from build123d import *

# Parameters (mm, degrees)
F1_DEPTH = 12
F2_DEPTH = 7


# Not quite as in the source:
# - a feature of the source that left no trace in its solid (it failed there, or was rolled back) is left out


with BuildPart() as f1:
    # F0 (on Front) → F1 (new body)
    with BuildSketch(Plane.XZ):
        with BuildLine():
            Line((70, 130), (70, 230))
            ThreePointArc((70, 230), (0, 300), (-70, 230))
            Line((-70, 230), (-70, 130))
            ThreePointArc((-70, 130), (0, 60), (70, 130))
        make_face()
        with BuildLine():
            Line((-65, 130), (-65, 230))
            ThreePointArc((-65, 230), (0, 295), (65, 230))
            Line((65, 230), (65, 130))
            ThreePointArc((65, 130), (0, 65), (-65, 130))
        make_face(mode=Mode.SUBTRACT)
        with BuildLine():
            ThreePointArc((65, 230), (0, 295), (-65, 230))
            Line((-65, 230), (-65, 130))
            ThreePointArc((-65, 130), (0, 65), (65, 130))
            Line((65, 130), (65, 230))
        make_face()
        with BuildLine():
            Line((-50, 130), (-50, 230))
            ThreePointArc((-50, 230), (0, 280), (50, 230))
            Line((50, 230), (50, 130))
            ThreePointArc((50, 130), (0, 80), (-50, 130))
        make_face(mode=Mode.SUBTRACT)
    extrude(amount=F1_DEPTH)

    # F0 (on Front) → F2 (cut)
    with BuildSketch(Plane.XZ):
        with BuildLine():
            ThreePointArc((65, 230), (0, 295), (-65, 230))
            Line((-65, 230), (-65, 130))
            ThreePointArc((-65, 130), (0, 65), (65, 130))
            Line((65, 130), (65, 230))
        make_face()
        with BuildLine():
            Line((-50, 130), (-50, 230))
            ThreePointArc((-50, 230), (0, 280), (50, 230))
            Line((50, 230), (50, 130))
            ThreePointArc((50, 130), (0, 80), (-50, 130))
        make_face(mode=Mode.SUBTRACT)
    extrude(amount=F2_DEPTH, mode=Mode.SUBTRACT)


solid = f1.part
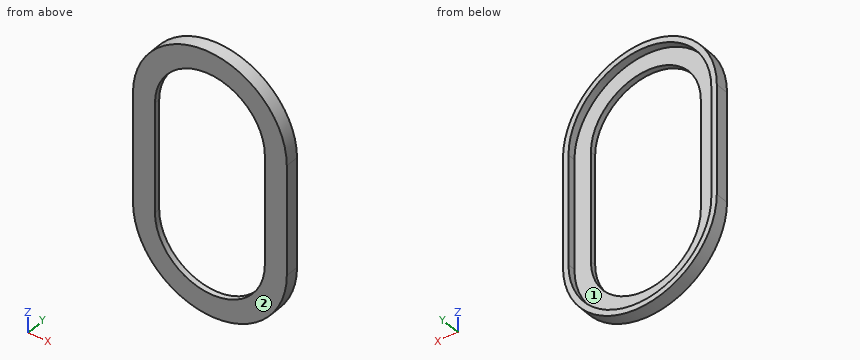
Geometry check sheet. Reference: the model listing, model coordinates, mm. Face numbers are marked on the shaded views. A direction names the side the tool comes from. Round coordinates to 2 decimals unless told otherwise and drop trailing zeros. Order: outer loops, then holes, each group sorted by start corner. A loop starts at its lowest first (then second) coordinate and runs counter-clockwise, first axis right, second up. Notation, with made-up numbers: (63.5, 19.25) -> (94.5, 19.25) arc R12 ccw to (94.5, 26.25) -> close; hole circle Ø2 at (11, 84.25). An arc over 180 degrees is marked (long way). Use one line per item in the form item = value.
1. Cross-section at C-C, the plane x = -56. Enter the section's corners in (y, z), plus the area to 3 significant figures.
Working result:
outline = (-12, 88) -> (0, 88) -> (0, 97) -> (-7, 97) -> (-7, 263) -> (0, 263) -> (0, 272) -> (-12, 272) -> close
area = 1,050 mm^2
2. Go/stop test with flat-tipped pins: pin 1 (6 mm diameter, centred on x = 35.5, y = -2, fed in from -Z); pin 2 (4 mm diameter, centred on y = -8, z = 258, fed in from -X); pin 3 (10 mm diameter, centred on x = -48.5, z = 128, fed in from +Y). Record where each tip stops, or that it passes through.
Working result:
pin_1 = 68
pin_2 = -64.99
pin_3 = -7
3. Scan lines: line 1 along X through (y, z) = (-0.5, 173); line 2 along X through (y, z) = (-9.5, 138.5); line 3 along Y through (x, z) = (57, 141.5). Record each from-to range of solid material in increasing order. Write a range as from..to.
Working result:
line_1 = -70..-65, 65..70
line_2 = -70..-50, 50..70
line_3 = -12..-7
4. Set-up check for the marked faces 1 and 2: record each of +Z, -Z, +X, -X, +Y, -Y from which the full face is reachable in a straight line by a thin tool's end or side.
Working result:
face_1 = +Y
face_2 = +Z, -Z, +X, -X, -Y
5. Cross-section at B-B, the plane z = 239. Enter the section's corners in (x, y).
Working result:
outline = (-69.42, -12) -> (-49.18, -12) -> (-49.18, -7) -> (-64.37, -7) -> (-64.37, 0) -> (-69.42, 0) -> close; (49.18, -12) -> (69.42, -12) -> (69.42, 0) -> (64.37, 0) -> (64.37, -7) -> (49.18, -7) -> close
6. Cross-section at D-D, the plane x = 53.5. Enter the section's corners in (y, z), plus the area to 3 significant figures.
Working result:
outline = (-12, 84.86) -> (0, 84.86) -> (0, 93.08) -> (-7, 93.08) -> (-7, 266.92) -> (0, 266.92) -> (0, 275.14) -> (-12, 275.14) -> close
area = 1,070 mm^2
7. Cross-section at A-A, the plane x = 0. Enter the section's corners in (y, z), plus the area to 3 significant figures.
Working result:
outline = (-12, 60) -> (0, 60) -> (0, 65) -> (-7, 65) -> (-7, 80) -> (-12, 80) -> close; (-12, 280) -> (-7, 280) -> (-7, 295) -> (0, 295) -> (0, 300) -> (-12, 300) -> close
area = 270 mm^2
